from build123d import *

# Parameters (mm, degrees)
PAD_DEPTH    = 20
SKETCH001_R  = 2.6
POCKET_DEPTH = 10.251
FILLET_R     = 1


with BuildPart() as part:
    # Sketch → Pad (new body)
    with BuildSketch(Plane.XY):
        with BuildLine():
            ThreePointArc((-1.5, 1.5), (0, 0), (1.5, 1.5))
            Line((1.5, 1.5), (1.5, 46.5))
            ThreePointArc((1.5, 46.5), (2.745624, 48.649808), (1.75, 50.926206))
            Line((1.75, 50.926206), (1.75, 54.282112))
            ThreePointArc((4.5, 45.225431), (5.501953, 50.475517), (1.75, 54.282112))
            Line((4.5, 45.225431), (4.5, 0.225431))
            ThreePointArc((-4.5, 0.225431), (0, -3.177021), (4.5, 0.225431))
            Line((-4.5, 0.225431), (-4.5, 45.225431))
            ThreePointArc((-1.75, 54.282112), (-5.501953, 50.475517), (-4.5, 45.225431))
            Line((-1.75, 54.282112), (-1.75, 50.926206))
            ThreePointArc((-1.75, 50.926206), (-2.745624, 48.649808), (-1.5, 46.5))
            Line((-1.5, 1.5), (-1.5, 46.5))
        make_face()
    extrude(amount=PAD_DEPTH)

    # Sketch001 (on Face6 of Pad) → Pocket (cut, through all)
    with BuildSketch(Plane.YZ.offset(4.5)):
        with Locations((22.5, 10)):
            Circle(SKETCH001_R)
    extrude(amount=-POCKET_DEPTH, mode=Mode.SUBTRACT)

    # Fillet
    fillet_edges = [part.edges().sort_by_distance(p)[0] for p in [
        (-1.75, 54.282112, 10),
        (1.75, 54.282112, 10),
    ]]
    fillet(fillet_edges, radius=FILLET_R)


solid = part.part
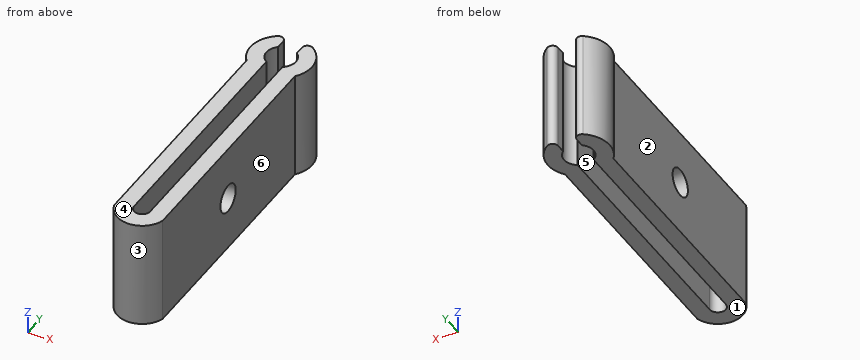
Model file for the job. Use its own axes, mm. Face numbers are marked on the shaded views. A direction names the side the tool comes from. Coordinates: 2 decimals unless noted, no trailing zeros. Write each loop counter-clockwise with the first axis right and the second up, starting at its lowest first coordinate (ties: lowest second). Pieces come first, ordered by that corner, then holes. Notation, with made-up numbers: (-3.5, 20.5) -> (4.5, 20.5) arc R31 ccw to (4.5, 49.5) -> close; hole circle Ø4 at (0.25, 35). An arc over 180 degrees is marked (long way). One line per item, written item: value. Start each with the question number.
1) Flat gauge pins, fed straight in: pin 1 Ø0.9 at (y, z) = (52, 13.5) entering from +X; pin 2 Ø8.5 at (y, z) = (22.5, 10) entering from -X; pin 3 Ø4 at (x, z) = (-2.5, 4) entering from -Y; pin 4 Ø3 at (x, z) = (3, 11.5) entering from +Y. Where does each tip first touch, or does it go through?
2) Which spindle directions (+Z, -Z, +X, -X, +Y, -Y) get a long thin tool onto all of the face, cutting with end or side? Do the marked faces 1 and 2. Say none if no direction does.
3) Slice it at A-A on y = 22.5. Write the cut outline in (x, z), then the cut area to 3 significant figures.
4) Slice it at D-D on z = 2. Write the cut outline in (x, y), then the cut area to 3 significant figures.
5) Pull direction X, two halves, no side cores. Call the marked faces 3, 4, 5 and 6: +X half, -X half, draft (parallel to the pull), parting line (faces both ways), or undercut.
6) Probe probe 1 along Z at (x, y) = (-2.9, 22.5); probe 2 along X at (y, z) = (8.5, 17); probe 3 along X at (y, z) = (46.5, 14.25). List the from-to ranges inside material, lowest first.
7) Slice it at C-C on y = 29. Write the cut outline in (x, z).
8) Slice it at B-B on z = 10. Write the cut outline in (x, y).
Answers follow:
1. pin 1: x = 5.05
1. pin 2: x = -4.5
1. pin 3: y = -3.15
1. pin 4: y = 53.68
2. face 1: -Z, +X, -X, +Y, -Y
2. face 2: +Z, -Z, -X, -Y
3. outline: (-4.5, 0) -> (-1.5, 0) -> (-1.5, 7.4) -> (-4.5, 7.4) -> close; (-4.5, 12.6) -> (-1.5, 12.6) -> (-1.5, 20) -> (-4.5, 20) -> close; (1.5, 0) -> (4.5, 0) -> (4.5, 7.4) -> (1.5, 7.4) -> close; (1.5, 12.6) -> (4.5, 12.6) -> (4.5, 20) -> (1.5, 20) -> close
3. area: 88.8 mm2
4. outline: (-4.5, 0.23) arc R4.68 ccw to (4.5, 0.23) -> (4.5, 45.23) arc R5.75 ccw to (3.33, 53.49) arc R1 ccw to (1.75, 52.68) -> (1.75, 50.93) arc R2.75 cw to (1.5, 46.5) -> (1.5, 1.5) arc R1.5 cw to (-1.5, 1.5) -> (-1.5, 46.5) arc R2.75 cw to (-1.75, 50.93) -> (-1.75, 52.68) arc R1 ccw to (-3.33, 53.49) arc R5.75 ccw to (-4.5, 45.23) -> close
4. area: 344 mm2
5. face 3: parting line
5. face 4: draft
5. face 5: undercut
5. face 6: +X half
6. probe 1: 0 to 7.4, 12.6 to 20
6. probe 2: -4.5 to -1.5, 1.5 to 4.5
6. probe 3: -5.27 to -1.5, 1.5 to 5.27
7. outline: (-4.5, 0) -> (-1.5, 0) -> (-1.5, 20) -> (-4.5, 20) -> close; (1.5, 0) -> (4.5, 0) -> (4.5, 20) -> (1.5, 20) -> close
8. outline: (-4.5, 0.23) arc R4.68 ccw to (4.5, 0.23) -> (4.5, 19.9) -> (1.5, 19.9) -> (1.5, 1.5) arc R1.5 cw to (-1.5, 1.5) -> (-1.5, 19.9) -> (-4.5, 19.9) -> close; (-4.5, 25.1) -> (-1.5, 25.1) -> (-1.5, 46.5) arc R2.75 cw to (-1.75, 50.93) -> (-1.75, 52.68) arc R1 ccw to (-3.33, 53.49) arc R5.75 ccw to (-4.5, 45.23) -> close; (1.5, 25.1) -> (4.5, 25.1) -> (4.5, 45.23) arc R5.75 ccw to (3.33, 53.49) arc R1 ccw to (1.75, 52.68) -> (1.75, 50.93) arc R2.75 cw to (1.5, 46.5) -> close
